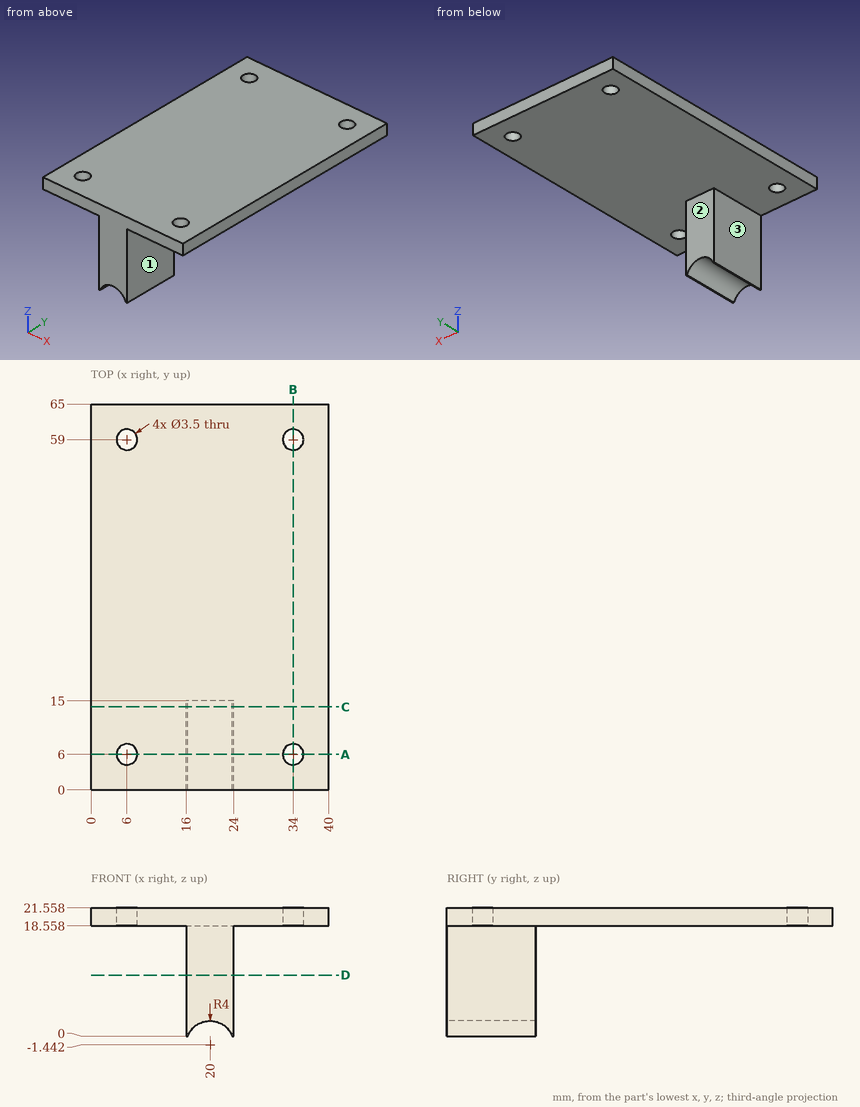
Study the drawing (mm; zero at the part's minimum x, y, z) and answer. A direction names the side the tool comes from. Coordinates: 2 decimals unless noted, no trailing zeros. Order: outer loops, then holes, each group sorted by start corner. A loop starts at its lowest first (then second) coordinate and runs counter-clockwise, first axis right, second up. Notation, with made-up numbers: M 76.5,21.5 L 89.5,21.5 A21 cw 89.5,34.5 Z; hole C -12.75,11 d11. An arc over 180 degrees is marked long. Answer as a JSON object with one key per item and string values. Group by question number.
1. Section A-A on y = 6 is taken. Write down the section's boundary in (x, z).
2. Section B-B on x = 34 is taken. Write down the section's boundary in (y, z), then the cut area to 3 significant figures.
3. Section C-C on y = 14 is taken. Write down the section's boundary in (x, z), then the cut area to 3 significant figures.
4. Straight lines are drawn through the part: line 1 (Y direction, x = 6, z = 19.45); line 2 (Z direction, x = 13, y = 19); line 3 (X direction, y = 5, z = 14.5). For each, find the intervals that lie inside material, in ascending order.
5. A tool of negligible diameter and unlimited length cuts with its end or side. For the marked faces 1, 2 and 3, from which of +Z, -Z, +X, -X, +Y, -Y can it reach the whole face along a straight path? Write none if from no direction.
6. Section D-D on z = 10.25 is taken. Write down the section's boundary in (x, y), then the cut area to 3 significant figures.
7. Flat-ended cylindrical pins translate along their axes: P1, Ø2, axis at x = 34, y = 6, coming from the +Z side; P2, Ø4.5, axis at x = 6, y = 59, coming from the -Z side; P3, Ø2, axis at x = 20, z = 12.5, coming from the +Y side; P4, Ø4.5, axis at y = 6.5, z = 5.5, coming from the +X side. Find the tip coordinate at first contact, or state that the pin passes through.
Values follow:
{
 "1": {"outline": "M 0,18.56 L 4.25,18.56 L 4.25,21.56 L 0,21.56 Z; M 7.75,18.56 L 16,18.56 L 16,0 L 16.27,0 A4 cw 23.73,0 L 24,0 L 24,18.56 L 32.25,18.56 L 32.25,21.56 L 7.75,21.56 Z; M 35.75,18.56 L 40,18.56 L 40,21.56 L 35.75,21.56 Z"},
 "2": {"outline": "M 0,18.56 L 4.25,18.56 L 4.25,21.56 L 0,21.56 Z; M 7.75,18.56 L 57.25,18.56 L 57.25,21.56 L 7.75,21.56 Z; M 60.75,18.56 L 65,18.56 L 65,21.56 L 60.75,21.56 Z", "area": "174 mm2"},
 "3": {"outline": "M 0,18.56 L 16,18.56 L 16,0 L 16.27,0 A4 cw 23.73,0 L 24,0 L 24,18.56 L 40,18.56 L 40,21.56 L 0,21.56 Z", "area": "255 mm2"},
 "4": {"line 1": "0 to 4.25, 7.75 to 57.25, 60.75 to 65", "line 2": "18.56 to 21.56", "line 3": "16 to 24"},
 "5": {"face 1": "-Z, +X, +Y, -Y", "face 2": "-Z, +X, -X, +Y", "face 3": "-Z, -X, +Y, -Y"},
 "6": {"outline": "M 16,0 L 24,0 L 24,15 L 16,15 Z", "area": "120 mm2"},
 "7": {"P1": "through", "P2": "z = 18.56", "P3": "y = 15", "P4": "x = 24"}
}
